```python
from build123d import *

# Parameters (mm, degrees)
F0_R     = 32.815242
F1_DEPTH = 76.2
F2_R     = 5.08
F3_R     = 26.928884
F4_DEPTH = 50.8


with BuildPart() as f1:
    # F0 (on Top) → F1 (new body)
    with BuildSketch(Plane.XY):
        Circle(F0_R)
    extrude(amount=F1_DEPTH)

    # F2
    f2_edges = [f1.edges().sort_by_distance(p)[0] for p in [
        (-32.815242, 0, 76.2),
    ]]
    fillet(f2_edges, radius=F2_R)

    # F3 (on face) → F4 (cut)
    with BuildSketch(Plane(origin=(0, 0, 0), x_dir=(1, 0, 0), z_dir=(0, 0, -1))):
        Circle(F3_R)
    extrude(amount=-F4_DEPTH, mode=Mode.SUBTRACT)


solid = f1.part
```
Model file for the job. Use its own axes, mm. A direction names the side the tool comes from. Coordinates: 2 decimals unless noted, no trailing zeros. Loops run counter-clockwise (first coordinate to the right, second up) from the corner with the lowest first, then second, coordinate; pieces in that order, holes last. Notation, with made-up numbers: (-20.5, 84.25) - (20.5, 84.25) arc R27 ccw to (20.5, 109.25) - close; hole circle Ø2 at (7, 14.25). An arc over 180 degrees is marked (long way). Answer as a JSON object with one key per item and string values. Group by question number.
(1) Cut at A-A (x = 0). Give the cut face in (y, z), then the cut area to 3 significant figures.
(2) Two-plate mould, pull along Y, no slides. Class faces 1 (the face through (31.3, 9.86, 35.06)), 2 (the face through (0, 0, 50.8)), 3 (the face through (0, 0, 76.2)): released by +Y, released by -Y, zero draft, split by the parting line, or undercut.
(3) Probe line 1 along Y through (x, z) = (0, 35); line 2 along Z through (x, y) = (14, -21); line 3 along X through (y, z) = (3.5, 33). List the from-to ranges inside material, lowest first.
(4) Tool access for faces 4 (the face through (-26.903, -1.184, 25.044)), 5 (the face through (-3, 27, 0)): list every direction of +Z, -Z, +X, -X, +Y, -Y with a clear straight run to the whole face (end or side of a thin tool).
(5) Flat gauge pins, fed straight in: pin 1 (1 mm diameter, centred on y = 19, z = 48.5, fed in from +X); pin 2 (1.5 mm diameter, centred on x = 24.5, y = -8.5, fed in from -Z); pin 3 (6 mm diameter, centred on y = 18.5, z = 63.5, fed in from -X). Where does each tip first touch, or does it go through?
(6) Cut at C-C (z = 6.5). Give the cut face in (x, y), then the cut area to 3 significant figures.
Geometry says:
{
 "1": {"outline": "(-32.82, 0) - (-26.93, 0) - (-26.93, 50.8) - (26.93, 50.8) - (26.93, 0) - (32.82, 0) - (32.82, 71.12) arc R5.08 ccw to (27.74, 76.2) - (-27.74, 76.2) arc R5.08 ccw to (-32.82, 71.12) - close", "area": "2,250 mm^2"},
 "2": {"face 1": "split by the parting line", "face 2": "undercut", "face 3": "zero draft"},
 "3": {"line 1": "y = -32.82 to -26.93, 26.93 to 32.82", "line 2": "z = 50.8 to 76.2", "line 3": "x = -32.63 to -26.7, 26.7 to 32.63"},
 "4": {"face 4": "-Z", "face 5": "-Z, +X, -X, +Y, -Y"},
 "5": {"pin 1": "stops at x = 27.1", "pin 2": "stops at z = 50.8", "pin 3": "stops at x = -28.92"},
 "6": {"outline": "circle Ø65.63 at (0, 0); hole circle Ø53.86 at (0, 0)", "area": "1,100 mm^2"}
}
